Part model, mm, in its own coordinate system. Round coordinates to 2 decimals unless told otherwise and drop trailing zeros. Loops run counter-clockwise (first coordinate to the right, second up) from the corner with the lowest first, then second, coordinate; pieces in that order, holes last. Notation, with made-up numbers: (47, -38) -> (79, -38) arc R25 cw to (79, -26) -> close; hole circle Ø3 at (22.25, 21.5). An arc over 180 degrees is marked (long way). Answer as CSV lines item,"result".
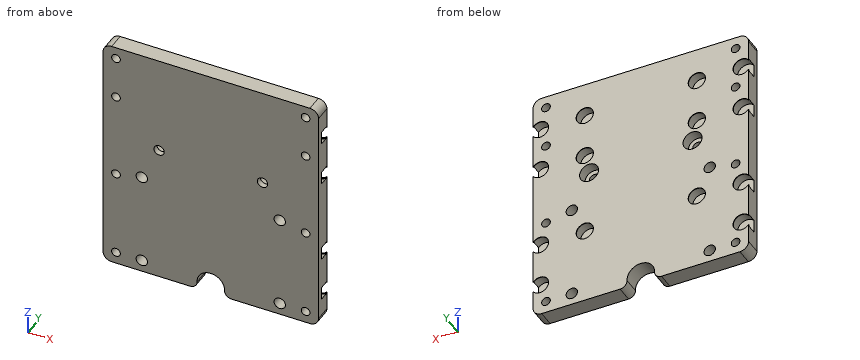
Autodesk Fusion 360 part; units mm, degrees
sketch "Sketch1" plane through (0, 0, 0) normal (0, 1, 0) x (1, 0, 0)
  line L0 (22.5, -7) -> (22.5, -61) construction
  line L1 (121, -45) -> (121, -19) construction
  line L2 (95, -120) -> (121, -120) construction
  line L3 (22.5, -61) -> (102.5, -61) construction
  line L4 (102.5, -61) -> (102.5, -7) construction
  line L5 (95, -94) -> (95, -120) construction
  line L6 (30, -19) -> (4, -19) construction
  line L7 (121, -19) -> (95, -19) construction
  line L8 (32.5, -82) -> (92.5, -82) construction
  line L9 (125, 0) -> (74.4896, 0)
  line L10 (4, -45) -> (30, -45) construction
  arc A0 (54.5069, -4.1667) -> (70.4931, -4.1667) centre (62.5, -4.5) ccw
  line L11 (50.5104, 0) -> (0, 0)
  line L12 (4, -120) -> (30, -120) construction
  line L13 (30, -94) -> (4, -94) construction
  line L14 (102.5, -7) -> (22.5, -7) construction
  arc A1 (74.4896, 0) -> (70.4931, -4.1667) centre (74.4896, -4) ccw
  arc A2 (54.5069, -4.1667) -> (50.5104, 0) centre (50.5104, -4) ccw
  line L15 (30, -120) -> (30, -94) construction
  line L16 (95, -45) -> (121, -45) construction
  line L17 (125, -140) -> (125, 0)
  line L18 (4, -94) -> (4, -120) construction
  line L19 (95, -19) -> (95, -45) construction
  line L20 (121, -94) -> (95, -94) construction
  line L21 (4, -19) -> (4, -45) construction
  line L22 (121, -120) -> (121, -94) construction
  line L23 (30, -45) -> (30, -19) construction
  line L24 (0, -140) -> (125, -140)
  line L25 (62.5, -140) -> (62.5, 80) construction
  line L26 (0, 0) -> (0, -140)
  dimension "d19" = 26
  dimension "d20" = 26
  dimension "d21" = 26
  dimension "d22" = 20
  dimension "d23" = 140
  dimension "d55" = 40
  dimension "d56" = 40
  dimension "d28" = 49
  dimension "d29" = 54
  dimension "d34" = 82
  dimension "d36" = 16
  dimension "d37" = 4.5
  dimension "d39" = 8
  dimension "d44" = 125
  dimension "d45" = 65
  dimension "d46" = 32.5
  dimension "d47" = 60
  dimension "d50" = 30
  dimension "d51" = 7
extrude "Extrude1" add sketch "Sketch1" against normal blind 9.525
hole "Hole2" at (95, 0, 120) at (121, 0, 120) at (121, 0, 94) at (95, 0, 94) at (30, 0, 120) at (30, 0, 94) at (4, 0, 94) at (4, 0, 120) at (121, 0, 45) at (121, 0, 19) at (95, 0, 45) at (30, 0, 45) at (4, 0, 45) at (4, 0, 19) direction (0, -1, 0) diameter 11 depth 6.1 tip angle 180 counterbore diameter 10 counterbore depth 0.338
hole "Hole3" at (92.5, 0, 82) at (32.5, 0, 82) direction (0, -1, 0) diameter 6 depth 10 tip angle 180 counterbore diameter 11 counterbore depth 6.1
fillet "Fillet1" radius 5 4 edges at (125, -4.7625, 140) (125, -4.7625, 0) (0, -4.7625, 0) (0, -4.7625, 140)
sketch "Sketch4" plane through (0, 0, 0) normal (0, 1, 0) x (1, 0, 0)
  arc A0 (0, -135) -> (5, -140) centre (5, -135) ccw construction
  line L0 (0, -5) -> (0, -15.2251) construction
  arc A1 (5, 0) -> (0, -5) centre (5, -5) ccw construction
  line L1 (50.5104, 0) -> (5, 0) construction
  arc A2 (54.5069, -4.1667) -> (50.5104, 0) centre (50.5104, -4) ccw construction
  arc A3 (54.5069, -4.1667) -> (70.4931, -4.1667) centre (62.5, -4.5) ccw construction
  arc A4 (74.4896, 0) -> (70.4931, -4.1667) centre (74.4896, -4) ccw construction
  line L2 (120, 0) -> (74.4896, 0) construction
  arc A5 (125, -5) -> (120, 0) centre (120, -5) ccw construction
  line L3 (125, -135) -> (125, -123.7749) construction
  arc A6 (120, -140) -> (125, -135) centre (120, -135) ccw construction
  line L4 (5, -140) -> (120, -140) construction
  line L5 (7.5, -108) -> (117.5, -108) construction
  line L6 (117.5, -108) -> (117.5, -58) construction
  line L7 (117.5, -58) -> (7.5, -58) construction
  line L8 (7.5, -58) -> (7.5, -108) construction
  line L9 (62.5, -140) -> (62.5, -12.5) construction
  circle A7 centre (92.5, -82) radius 5.5
  circle A8 centre (32.5, -82) radius 5.5
  arc A9 (125, -116.2251) -> (125, -123.7749) centre (121, -120) ccw
  line L10 (125, -116.2251) -> (125, -97.7749)
  arc A10 (125, -90.2251) -> (125, -97.7749) centre (121, -94) ccw
  line L11 (125, -90.2251) -> (125, -48.7749)
  arc A11 (125, -41.2251) -> (125, -48.7749) centre (121, -45) ccw
  line L12 (125, -41.2251) -> (125, -22.7749)
  arc A12 (125, -15.2251) -> (125, -22.7749) centre (121, -19) ccw
  line L13 (125, -15.2251) -> (125, -5)
  arc A13 (0, -22.7749) -> (0, -15.2251) centre (4, -19) ccw
  line L14 (0, -22.7749) -> (0, -41.2251)
  arc A14 (0, -48.7749) -> (0, -41.2251) centre (4, -45) ccw
  line L15 (0, -48.7749) -> (0, -90.2251)
  arc A15 (0, -97.7749) -> (0, -90.2251) centre (4, -94) ccw
  line L16 (0, -97.7749) -> (0, -116.2251)
  arc A16 (0, -123.7749) -> (0, -116.2251) centre (4, -120) ccw
  line L17 (0, -123.7749) -> (0, -135)
  circle A17 centre (30, -45) radius 5.5
  circle A18 centre (30, -94) radius 5.5
  circle A19 centre (95, -94) radius 5.5
  circle A20 centre (95, -120) radius 5.5
  circle A21 centre (30, -120) radius 5.5
  circle A22 centre (95, -45) radius 5.5
  dimension "d73" = 110
  dimension "d74" = 55
  dimension "d76" = 32
  dimension "d90" = 50
hole "Hole1" at (7.5, 0, 108) at (7.5, 0, 58) at (117.5, 0, 108) at (117.5, 0, 58) direction (0, -1, 0) diameter 5.035 depth 10 tip angle 180
hole "Hole4" at (102.5, 0, 61) at (22.5, 0, 61) at (22.5, 0, 7) at (102.5, 0, 7) direction (0, -1, 0) diameter 6.6 depth 10 tip angle 180
sketch "Sketch5" plane through (0, -9.525, 0) normal (0, -1, 0) x (1, 0, 0)
  circle A0 centre (22.5, 7) radius 3.3
  circle A1 centre (102.5, 61) radius 3.3
  circle A2 centre (22.5, 61) radius 3.3
  circle A3 centre (102.5, 7) radius 3.3
  circle A4 centre (117.5, 108) radius 2.5175
  circle A5 centre (7.5, 108) radius 2.5175
  circle A6 centre (7.5, 58) radius 2.5175
  circle A7 centre (117.5, 58) radius 2.5175
  arc A8 (5, 140) -> (0, 135) centre (5, 135) ccw
  line L0 (0, 135) -> (0, 5)
  arc A9 (0, 5) -> (5, 0) centre (5, 5) ccw
  line L1 (5, 0) -> (50.5104, 0)
  arc A10 (50.5104, 0) -> (54.5069, 4.1667) centre (50.5104, 4) ccw
  arc A11 (70.4931, 4.1667) -> (54.5069, 4.1667) centre (62.5, 4.5) ccw
  arc A12 (70.4931, 4.1667) -> (74.4896, 0) centre (74.4896, 4) ccw
  line L2 (74.4896, 0) -> (120, 0)
  arc A13 (120, 0) -> (125, 5) centre (120, 5) ccw
  line L3 (125, 5) -> (125, 135)
  arc A14 (125, 135) -> (120, 140) centre (120, 135) ccw
  line L4 (120, 140) -> (5, 140)
  circle A15 centre (92.5, 82) radius 3
  circle A16 centre (32.5, 82) radius 3
  line L5 (0, 133) -> (125, 133) construction
  line L6 (62.5, 140) -> (62.5, 75.63) construction
  line L7 (7.5, 133) -> (117.5, 133)
  line L8 (117.5, 133) -> (117.5, 7)
  line L9 (117.5, 7) -> (7.5, 7)
  line L10 (7.5, 7) -> (7.5, 133)
  line L11 (7.5, 133) -> (117.5, 7) construction
  line L12 (117.5, 133) -> (7.5, 7) construction
  point P0 (7.5, 133)
  point P1 (117.5, 133)
  point P2 (62.5, 70)
  dimension "d94" = 55
  dimension "d95" = 110
  dimension "d96" = 7
  dimension "d100" = 7
hole "Hole5" at (7.5, -9.525, 133) at (117.5, -9.525, 133) at (117.5, -9.525, 7) at (7.5, -9.525, 7) direction (0, 1, 0) diameter 5.035 depth 35 tip angle 118
Q1. Saw through at A-A, the plane z = 133. Write the cut outline in (x, y) (1 decimal), then the cut area to 3 significant figures.
Geometry results:
outline,"(0, -9.5) -> (5, -9.5) -> (5, 0) -> (0, 0) -> close; (10, -9.5) -> (115, -9.5) -> (115, 0) -> (10, 0) -> close; (120, -9.5) -> (125, -9.5) -> (125, 0) -> (120, 0) -> close"
area,"1,090 mm2"
Q2. Saw through at D-D, the plane x = 61. Write the cut outline in (y, z) (3 decimals).
Geometry results:
outline,"(-9.525, 12.358) -> (0, 12.358) -> (0, 140) -> (-9.525, 140) -> close"
Q3. Drill centre lines: line 1 along X through (y, z) = (-2.5, 133); line 2 along X through (y, z) = (-0.15, 120); line 3 along Z through (x, y) = (4, -3.65). Where is each one in solid material? Low to high.
Geometry results:
line 1,"0 to 4.98, 10.02 to 114.98, 120.02 to 125"
line 2,"9 to 25, 35 to 90, 100 to 116"
line 3,"0.1 to 13.5, 24.5 to 39.5, 50.5 to 88.5, 99.5 to 114.5, 125.5 to 139.9"
Q4. Drop flat-ended pins along their axis: P1, Ø1.5, axis at x = 31, y = -7, coming from the -Z side; P2, Ø5, axis at x = 5, z = 119, coming from the +Y side; P3, Ø4, axis at x = 64.5, y = -2.5, coming from the -Z side; P4, Ø4, axis at x = 7.5, z = 58, coming from the -Y side. Give the stop position or say it passes through.
Geometry results:
P1,"z = 0"
P2,"y = -6.1"
P3,"z = 11.43"
P4,"through"
Q5. Saw through at C-C, the plane z = 94. Write the cut outline in (x, y) (3 decimals), then the cut area to 3 significant figures.
Geometry results:
outline,"(0, -9.525) -> (125, -9.525) -> (125, -6.1) -> (115.5, -6.1) -> (115.5, -0.338) -> (116, -0.338) -> (116, 0) -> (100, 0) -> (100, -0.338) -> (100.5, -0.338) -> (100.5, -6.1) -> (89.5, -6.1) -> (89.5, -0.338) -> (90, -0.338) -> (90, 0) -> (35, 0) -> (35, -0.338) -> (35.5, -0.338) -> (35.5, -6.1) -> (24.5, -6.1) -> (24.5, -0.338) -> (25, -0.338) -> (25, 0) -> (9, 0) -> (9, -0.338) -> (9.5, -0.338) -> (9.5, -6.1) -> (0, -6.1) -> close"
area,"942 mm2"
Q6. Saw through at B-B, the plane y = -7.75. Give the number of separate pieces and of enclosed holes in the cut face, then the cut area to 3 significant figures.
Geometry results:
separate pieces,"1"
enclosed holes,"14"
area,"16,900 mm2"
